```python
from build123d import *

# Parameters (mm, degrees)
BOSS_EXTRUDE1_DEPTH     = 3.175
CUT_EXTRUDE1_DEPTH      = 1
CUT_EXTRUDE1_DEPTH_BACK = 4.175
SKETCH4_R               = 2.413
CUT_EXTRUDE2_DEPTH      = 4.175
SKETCH5_R               = 2.5
SKETCH5_R_2             = 2.47796547
CUT_EXTRUDE3_DEPTH      = 4.175
SKETCH6_R               = 2.321781934
SKETCH6_R_2             = 3.272341149
SKETCH6_R_3             = 2.5
SKETCH6_R_4             = 1.905
SKETCH6_R_5             = 1.75
CUT_EXTRUDE4_DEPTH      = 4.175


with BuildPart() as part:
    # Sketch1 → Boss-Extrude1 (new body)
    with BuildSketch(Plane(origin=(0, 0, 0), x_dir=(1, 0, 0), z_dir=(0, 1, 0))):
        with BuildLine():
            Line((-127, -355.6), (127, -355.6))
            ThreePointArc((127, -355.6), (193.955389821, -193.955389821), (355.6, -127))
            Line((355.6, -127), (355.6, 127))
            ThreePointArc((355.6, 127), (193.955389821, 193.955389821), (127, 355.6))
            Line((127, 355.6), (-127, 355.6))
            ThreePointArc((-127, 355.6), (-193.955389821, 193.955389821), (-355.6, 127))
            Line((-355.6, 127), (-355.6, -127))
            ThreePointArc((-355.6, -127), (-193.955389821, -193.955389821), (-127, -355.6))
        make_face()
    extrude(amount=BOSS_EXTRUDE1_DEPTH)

    # Sketch2 → Cut-Extrude1 (cut, two sides)
    with BuildSketch(Plane(origin=(0, 3.175, 0), x_dir=(1, 0, 0), z_dir=(0, 1, 0))) as cut_extrude1_sk:
        with BuildLine():
            Line((-304.8, 2.413), (-293.37, 2.413))
            ThreePointArc((-293.37, 2.413), (-290.957, 0), (-293.37, -2.413))
            Line((-293.37, -2.413), (-304.8, -2.413))
            ThreePointArc((-304.8, -2.413), (-307.213, 0), (-304.8, 2.413))
        make_face()
        with BuildLine():
            Line((-304.8, -22.987), (-293.37, -22.987))
            ThreePointArc((-293.37, -22.987), (-290.957, -25.4), (-293.37, -27.813))
            Line((-293.37, -27.813), (-304.8, -27.813))
            ThreePointArc((-304.8, -27.813), (-307.213, -25.4), (-304.8, -22.987))
        make_face()
        with BuildLine():
            Line((-285.75, -2.413), (-274.32, -2.413))
            ThreePointArc((-274.32, -2.413), (-271.907, 0), (-274.32, 2.413))
            Line((-274.32, 2.413), (-285.75, 2.413))
            ThreePointArc((-285.75, 2.413), (-288.163, 0), (-285.75, -2.413))
        make_face()
        with BuildLine():
            Line((-285.75, -22.987), (-274.32, -22.987))
            ThreePointArc((-274.32, -22.987), (-271.907, -25.4), (-274.32, -27.813))
            Line((-274.32, -27.813), (-285.75, -27.813))
            ThreePointArc((-285.75, -27.813), (-288.163, -25.4), (-285.75, -22.987))
        make_face()
    extrude(amount=CUT_EXTRUDE1_DEPTH, mode=Mode.SUBTRACT)
    extrude(cut_extrude1_sk.sketch, amount=-CUT_EXTRUDE1_DEPTH_BACK, mode=Mode.SUBTRACT)

    # Sketch4 → Cut-Extrude2 (cut, through all)
    with BuildSketch(Plane(origin=(0, 3.175, 0), x_dir=(1, 0, 0), z_dir=(0, 1, 0))):
        with Locations((237.49, -9.430177049)):
            Circle(SKETCH4_R)
        with Locations((205.74, -9.430177049)):
            Circle(SKETCH4_R)
        with Locations((237.49, -39.910177049)):
            Circle(SKETCH4_R)
        with Locations((205.74, -39.910177049)):
            Circle(SKETCH4_R)
    extrude(amount=-CUT_EXTRUDE2_DEPTH, mode=Mode.SUBTRACT)

    # Sketch5 → Cut-Extrude3 (cut, through all)
    with BuildSketch(Plane.XZ):
        with Locations((-207.790149601, 50.01656837)):
            Circle(SKETCH5_R)
        with Locations((-206.624048203, -51.576739518)):
            Circle(SKETCH5_R)
        with Locations((8.09562966, 52.494533839)):
            Circle(SKETCH5_R_2)
        with Locations((9.261731058, -49.098774048)):
            Circle(SKETCH5_R)
    extrude(amount=-CUT_EXTRUDE3_DEPTH, mode=Mode.SUBTRACT)

    # Sketch6 → Cut-Extrude4 (cut, through all)
    with BuildSketch(Plane.XZ):
        with Locations((-131.96570437, 157.594741445)):
            Circle(SKETCH6_R)
        with Locations((-131.96570437, 106.794741445)):
            Circle(SKETCH6_R)
        with Locations((-178.700591901, 106.794741445)):
            Circle(SKETCH6_R)
        with Locations((-178.700591901, 157.594741445)):
            Circle(SKETCH6_R)
        with Locations((42.265908941, 162.337536061)):
            Circle(SKETCH6_R_2)
        with Locations((42.265908941, 86.137536061)):
            Circle(SKETCH6_R_3)
        with Locations((17.371687145, -109.265722508)):
            Circle(SKETCH6_R_4)
        with Locations((-25.681149945, -109.384160374)):
            Circle(SKETCH6_R_4)
        with Locations((-25.549785233, -157.135979683)):
            Circle(SKETCH6_R_4)
        with Locations((17.503045383, -157.015188359)):
            Circle(SKETCH6_R_4)
        with Locations((-84.882409293, -188.871278488)):
            Circle(SKETCH6_R_5)
        with Locations((-85.091846145, -164.872192335)):
            Circle(SKETCH6_R_5)
        with Locations((-116.881190831, -189.150527624)):
            Circle(SKETCH6_R_5)
        with Locations((-117.090627683, -165.151441471)):
            Circle(SKETCH6_R_5)
    extrude(amount=-CUT_EXTRUDE4_DEPTH, mode=Mode.SUBTRACT)


solid = part.part
```
Read the model definition and answer for the solid it produces. Units are mm, in the model's axes. Give positions to 0.01 mm unless a question says otherwise; leave off trailing zeros. Write each loop counter-clockwise with the first axis right and the second up, starting at its lowest first coordinate (ties: lowest second). Pieces come first, ordered by that corner, then holes. Notation, with made-up numbers: M 56,21.5 L 67,21.5 A12 cw 67,25.5 Z; hole C -13,-9 d9. An arc over 180 degrees is marked long. Put each result on its own line as item: value. Start each with the question number.
1. The part is cut by section A-A, the plane y = 2.1. Give the number of separate pieces and of enclosed holes in the cut face, and give its area (3 significant figures).
2. Consider line 1 along Z through (x, y) = (-300, 2.1); line 2 along X through (y, z) = (1.75, -50.5); line 3 along X through (y, z) = (1.15, -298). Determine where each line is inside the solid, lowest interval first.
3. The part is cut by section B-B, the plane x = -260. Give the vertices of the cut face in (y, z) (3 decimals).
4. Each of these flat-tipped pins is pushed along its axis until it touches: pin 1 Ø3 at (x, z) = (-85.09, -164.87) entering from -Y (3 decimals); pin 2 Ø1.6 at (x, y) = (-299, 2) entering from +Z; pin 3 Ø1.6 at (x, y) = (-297, 2.5) entering from -Z. Where does it stop, or does it pass through?
Final values:
1. separate pieces: 1
1. enclosed holes: 26
1. area: 341,000 mm²
2. line 1: z = -133.86 to -2.41, 2.41 to 22.99, 27.81 to 133.86
2. line 2: x = -355.6 to -208.88, -204.37 to 7.19, 11.33 to 355.6
2. line 3: x = -134.38 to 134.38
3. outline: M 0,-147.95 L 3.175,-147.95 L 3.175,147.95 L 0,147.95 Z
4. pin 1: passes through
4. pin 2: stops at z = 134.32
4. pin 3: stops at z = -134.85
